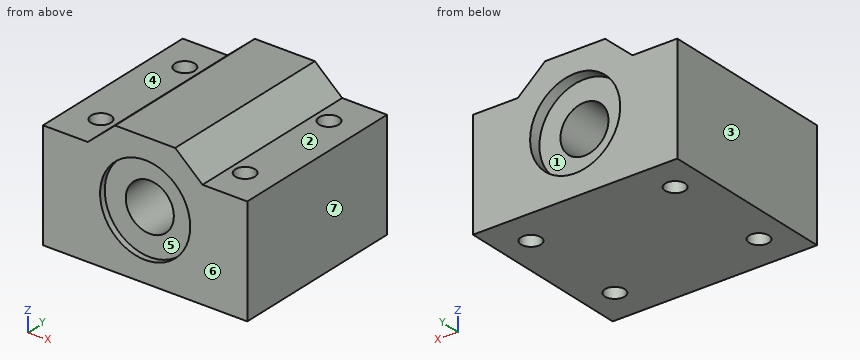
from build123d import *

# Parameters (mm, degrees)
F0_R     = 7.5
F1_DEPTH = 30
F2_START = -1
F0_R_2   = 4
F2_DEPTH = 27
F3_R     = 1.65
F4_DEPTH = 25


with BuildPart() as f1:
    # F0 (on Front) → F1 (new body)
    with BuildSketch(Plane.XZ):
        Polygon((-44, 18), (-44, 0), (-10, 0), (-10, 18), (-17.4580022789, 18), (-22, 22), (-32, 22), (-36.5419977211, 18), align=None)
        with Locations((-27, 11)):
            Circle(F0_R, mode=Mode.SUBTRACT)
    extrude(amount=-F1_DEPTH)

    # F0 (on Front) → F2 (join)
    with BuildSketch(Plane.XZ.offset(F2_START)):
        with Locations((-27, 11)):
            Circle(F0_R)
        with Locations((-27, 11)):
            Circle(F0_R_2, mode=Mode.SUBTRACT)
    extrude(amount=-F2_DEPTH)

    # F3 (on face) → F4 (cut)
    with BuildSketch(Plane(origin=(0, 0, 0), x_dir=(1, 0, 0), z_dir=(0, 0, -1))):
        with Locations((-39, -6)):
            Circle(F3_R)
        with Locations((-15, -6)):
            Circle(F3_R)
        with Locations((-15, -24)):
            Circle(F3_R)
        with Locations((-39, -24)):
            Circle(F3_R)
    extrude(amount=-F4_DEPTH, mode=Mode.SUBTRACT)


solid = f1.part
Design review of the part built by this model. Coordinates are the model's own, in mm. Face numbers are marked on the shaded views. A direction names the side the tool comes from. Round coordinates to 2 decimals unless told otherwise and drop trailing zeros. Write each loop counter-clockwise with the first axis right and the second up, starting at its lowest first coordinate (ties: lowest second). Pieces come first, ordered by that corner, then holes. Notation, with made-up numbers: (2.25, 5) - (49.25, 5) arc R25 ccw to (49.25, 32) - close; hole circle Ø1 at (-39, 54). An arc over 180 degrees is marked (long way). Return JSON: item names as keys, results as strings. Group by question number.
Item 1: For probe 1 along Y at (x, z) = (-15, 13.75); probe 2 along X at (y, z) = (6, 4.5); probe 3 along Z at (x, y) = (-27, 0.75), list the stretches that pass through material, from the lowest coordinate up. Write a range as [from, to].
Item 2: Machinability: for the marked faces 1, 2, 3 and 4, which of the approach directions +Z, -Z, +X, -X, +Y, -Y give a long, thin tool a straight path to every point of the face, cutting with its end or side? Answer none if there is none.
Item 3: We need section D-D on x = -15. Write out the cut boundary in (y, z).
Item 4: We need section A-A on z = 11. Write out the cut boundary in (x, y), and give its area (3 significant figures).
Item 5: We need section B-B on y = 24. Write out the cut boundary in (x, z), and give its area (3 significant figures).
Item 6: The part is to be moulded in two halves that separate along X. For the marked faces 5, 6 and 7, say which applies: pulls with the +X half, pulls with the -X half, needs draft (parallel to the pull), parting line crosses it, or undercut.
Item 7: We need section C-C on x = -27. Write out the cut boundary in (y, z).
Item 8: Insertion check: P1, Ø8, axis at x = -15.5, y = 16, coming from the +Z side; P2, Ø7.5, axis at x = -27, z = 11, coming from the +Y side; P3, Ø1.5, axis at x = -24, z = 17, coming from the +Y side; P4, Ø6, axis at x = -39.5, y = 19.5, coming from the +Z side. Each pin has a flat end and moves straight along its axis. Give the tip position at first contact, or say it passes through.
Model answer:
{
 "1": {"probe 1": "y = [0, 4.35], [7.65, 22.35], [25.65, 30]", "probe 2": "x = [-44, -40.65], [-37.35, -16.65], [-13.35, -10]", "probe 3": "z = [0, 3.5], [18.5, 22]"},
 "2": {"face 1": "+Y", "face 2": "+Z, +X, +Y, -Y", "face 3": "+Z, -Z, -X, +Y, -Y", "face 4": "+Z, -X, +Y, -Y"},
 "3": {"outline": "(0, 0) - (4.35, 0) - (4.35, 18) - (0, 18) - close; (7.65, 0) - (22.35, 0) - (22.35, 18) - (7.65, 18) - close; (25.65, 0) - (30, 0) - (30, 18) - (25.65, 18) - close"},
 "4": {"outline": "(-44, 0) - (-34.5, 0) - (-34.5, 1) - (-31, 1) - (-31, 28) - (-34.5, 28) - (-34.5, 30) - (-44, 30) - close; (-23, 1) - (-19.5, 1) - (-19.5, 0) - (-10, 0) - (-10, 30) - (-19.5, 30) - (-19.5, 28) - (-23, 28) - close; hole circle Ø3.3 at (-39, 6); hole circle Ø3.3 at (-39, 24); hole circle Ø3.3 at (-15, 6); hole circle Ø3.3 at (-15, 24)", "area": "725 mm²"},
 "5": {"outline": "(-44, 0) - (-40.65, 0) - (-40.65, 18) - (-44, 18) - close; (-37.35, 0) - (-16.65, 0) - (-16.65, 18) - (-17.46, 18) - (-22, 22) - (-32, 22) - (-36.54, 18) - (-37.35, 18) - close; (-13.35, 0) - (-10, 0) - (-10, 18) - (-13.35, 18) - close; hole circle Ø8 at (-27, 11)", "area": "501 mm²"},
 "6": {"face 5": "undercut", "face 6": "needs draft", "face 7": "pulls with the +X half"},
 "7": {"outline": "(0, 0) - (30, 0) - (30, 3.5) - (28, 3.5) - (28, 7) - (1, 7) - (1, 3.5) - (0, 3.5) - close; (0, 18.5) - (1, 18.5) - (1, 15) - (28, 15) - (28, 18.5) - (30, 18.5) - (30, 22) - (0, 22) - close"},
 "8": {"P1": "stops at z = 19.8", "P2": "passes through", "P3": "stops at y = 28", "P4": "stops at z = 18.04"}
}
